```python
from build123d import *

# Parameters (mm, degrees)
HEAD_DEPTH         = 12.7
HOLE_SKETCH_R      = 6.096
THROUGH_HOLE_DEPTH = 21.266683312


with BuildPart() as part:
    # Head Sketch → Head (new body)
    with BuildSketch(Plane.XY):
        Polygon((0, 10.558581723), (9.144, 5.279290861), (9.144, -5.279290861), (0, -10.558581723), (-9.144, -5.279290861), (-9.144, 5.279290861), align=None)
    extrude(amount=HEAD_DEPTH)

    # Flange Sketch → Flange (revolve)
    with BuildSketch(Plane(origin=(0, 0, 0), x_dir=(-1, 0, 0), z_dir=(0, 1, 0)), mode=Mode.PRIVATE) as flange_sk:
        with BuildLine():
            Line((-10.668, 0), (0, 0))
            Line((0, 0), (0, 3.81))
            ThreePointArc((0, 3.81), (-5.643297007, 3.079227926), (-10.91431477, 0.935119563))
            ThreePointArc((-10.91431477, 0.935119563), (-11.151507901, 0.372641807), (-10.668, 0))
        make_face()
    revolve(flange_sk.sketch.rotate(Axis((0, 0, 1.843425858), (0, 0, 1)), 30), axis=Axis((0, 0, 1.843425858), (0, 0, 1)))

    # Sketch5 → Head Trim (revolve, cut)
    with BuildSketch(Plane(origin=(0, 0, 0), x_dir=(0, 0, -1), z_dir=(1, 0, 0)), mode=Mode.PRIVATE) as head_trim_sk:
        with BuildLine():
            Line((-12.7, -8.018581723), (-12.7, -10.558581723))
            Line((-12.7, -10.558581723), (-10.16, -10.558581723))
            ThreePointArc((-10.16, -10.558581723), (-11.956051224, -9.814632947), (-12.7, -8.018581723))
        make_face()
    revolve(head_trim_sk.sketch.rotate(Axis((0, 0, 15.085599173), (0, 0, -1)), 90), axis=Axis((0, 0, 15.085599173), (0, 0, -1)), mode=Mode.SUBTRACT)

    # Hole Sketch → Through Hole (cut, through all)
    with BuildSketch(Plane.XY.offset(12.7)):
        Circle(HOLE_SKETCH_R)
    extrude(amount=-THROUGH_HOLE_DEPTH, mode=Mode.SUBTRACT)


solid = part.part
```
Can you work these out from the model? Positions are in its coordinate system, mm. A direction names the side the tool comes from. Coordinates: 2 decimals unless noted, no trailing zeros. Loops run counter-clockwise (first coordinate to the right, second up) from the corner with the lowest first, then second, coordinate; pieces in that order, holes last. Notation, with made-up numbers: (-15, 33) - (33, 33) arc R17 ccw to (33, 63) - close; hole circle Ø7 at (-2.5, -5). An arc over 180 degrees is marked (long way). Use a Markdown table: item, result.
Item 1: I want a section at C-C on z = 1.5. Please give me the cut outline in (x, y).
Numbers:
| item | result |
|---|---|
| outline | (-9.14, -5.28) - (-7.74, -6.09) arc R9.85 ccw to (-1.4, -9.75) - (0, -10.56) - (1.4, -9.75) arc R9.85 ccw to (7.74, -6.09) - (9.14, -5.28) - (9.14, -3.66) arc R9.85 ccw to (9.14, 3.66) - (9.14, 5.28) - (7.74, 6.09) arc R9.85 ccw to (1.4, 9.75) - (0, 10.56) - (-1.4, 9.75) arc R9.85 ccw to (-7.74, 6.09) - (-9.14, 5.28) - (-9.14, 3.66) arc R9.85 ccw to (-9.14, -3.66) - close; hole circle Ø12.19 at (0, 0) |
Item 2: We'd pull the mould along X, two halves only. Please class faces 1 (the face through (-0.794, 6.044, 6.439)), 2 (the face through (-2, 6, 12.7)), 3 (the face through (9.144, 0, 7)), 4 (the face through (-4.64, 7.88, 6.71)): released by +X, released by -X, zero draft, split by the parting line, or undercut.
Numbers:
| item | result |
|---|---|
| face 1 | undercut |
| face 2 | zero draft |
| face 3 | released by +X |
| face 4 | released by -X |
Item 3: Will these pins go through, and if not, where does the flat tip stop? pin 1 (4 mm diameter, centred on y = -4, z = 7.5, fed in from -X); pin 2 (1 mm diameter, centred on x = 0, y = 5, fed in from +Z); pin 3 (1 mm diameter, centred on x = -4.5, z = 2.5, fed in from -Y).
Numbers:
| item | result |
|---|---|
| pin 1 | stops at x = -9.14 |
| pin 2 | passes through |
| pin 3 | stops at y = -8.25 |
Item 4: For faces 5 (the face through (4.508, 7.956, 6.709)), 6 (the face through (6, -2, 0)), 7 (the face through (4.64, -7.88, 6.71)), 8 (the face through (-4.508, -7.956, 6.709)), which set-ups out of +Z, -Z, +X, -X, +Y, -Y let a thin tool reach every point of the face, with its end or its side?
Numbers:
| item | result |
|---|---|
| face 5 | +Z, +X, +Y |
| face 6 | -Z, +X, -X, +Y, -Y |
| face 7 | +Z, +X, -Y |
| face 8 | +Z, -X, -Y |
Item 5: I want a section at A-A on z = 5.5. Please give me the cut outline in (x, y), and give its area (3 significant figures).
Numbers:
| item | result |
|---|---|
| outline | (-9.14, -5.28) - (0, -10.56) - (9.14, -5.28) - (9.14, 5.28) - (0, 10.56) - (-9.14, 5.28) - close; hole circle Ø12.19 at (0, 0) |
| area | 173 mm2 |
Item 6: I want a section at D-D on z = 11.5. Please give me the cut outline in (x, y), and give its area (3 significant figures).
Numbers:
| item | result |
|---|---|
| outline | (-9.14, -4.47) arc R10.18 ccw to (-8.44, -5.69) - (-0.7, -10.15) arc R10.18 ccw to (0.7, -10.15) - (8.44, -5.69) arc R10.18 ccw to (9.14, -4.47) - (9.14, 4.47) arc R10.18 ccw to (8.44, 5.69) - (0.7, 10.15) arc R10.18 ccw to (-0.7, 10.15) - (-8.44, 5.69) arc R10.18 ccw to (-9.14, 4.47) - close; hole circle Ø12.19 at (0, 0) |
| area | 171 mm2 |
Item 7: If I drill on probe 1 along X at (y, z) = (-0.25, 10.75); probe 2 along Y at (x, z) = (2.5, 10.5); probe 3 along X at (y, z) = (1.5, 6.5), over which ranges is the centre line in solid material (lowest first)? Write a range as from..to.
Numbers:
| item | result |
|---|---|
| probe 1 | x = -9.14..-6.09, 6.09..9.14 |
| probe 2 | y = -9.12..-5.56, 5.56..9.12 |
| probe 3 | x = -9.14..-5.91, 5.91..9.14 |
Item 8: I want a section at B-B on y = 0. Please give me the cut outline in (x, z) (3 decimals).
Numbers:
| item | result |
|---|---|
| outline | (-10.914, 0.935) arc R0.5 ccw to (-10.668, 0) - (-6.096, 0) - (-6.096, 12.7) - (-8.019, 12.7) arc R2.54 ccw to (-9.144, 12.437) - (-9.144, 1.835) arc R22.155 ccw to start; (6.096, 0) - (10.668, 0) arc R0.5 ccw to (10.914, 0.935) arc R22.155 ccw to (9.144, 1.835) - (9.144, 12.437) arc R2.54 ccw to (8.019, 12.7) - (6.096, 12.7) - close |
